Autodesk Fusion 360 part; units mm, degrees
sketch "Sketch1" plane through (0, 0, 0) normal (0, 1, 0) x (1, 0, 0)
  circle A0 centre (0, 0) radius 20
  circle A1 centre (0, 0) radius 17
  dimension "d1" = 40
  dimension "d7" = 3
extrude "Extrude1" add sketch "Sketch1" along normal blind 70 makes body 1
extrude "Extrude2" add sketch "Sketch1" along normal blind 4 contours A1 bodies 1
copy_body "Body->Comp1" bodies 1 removing the originals makes body 2 in component "tubeToolHolder02"
component "tubeToolHolder02" placed x (1, 0, 0) y (0, 1, 0) z (0, 0, 1) at (0, 0, 0)
Read the model definition and answer for the solid it produces. Units are mm, in the model's axes. A direction names the side the tool comes from. Round coordinates to 2 decimals unless told otherwise and drop trailing zeros. Write each loop counter-clockwise with the first axis right and the second up, starting at its lowest first coordinate (ties: lowest second). Pieces come first, ordered by that corner, then holes. Notation, with made-up numbers: (87, 46) -> (139, 46) arc R18 cw to (139, 59) -> close; hole circle Ø2 at (13, 85.25). An arc over 180 degrees is marked (long way). Answer in a Markdown table with one row per item. Add a question column.
1) Find section A-A, the plane z = 0. Determine the outline of the cut face in (x, y), and give its area (3 significant figures).
2) Which of the six approach directions +Z, -Z, +X, -X, +Y, -Y give full straight-line access (tool end or side, diameter ignored) to faces 4 (the face through (-9, 70, 15)), 5 (the face through (0, 4, 0))?
3) Given P1, Ø1, axis at x = -6, y = 9, coming from the -Z side; P2, Ø4, axis at y = 29, z = -10, coming from the -X side; P3, Ø17, axis at x = -4, z = 0.5, coming from the +Y side, each flat-ended and moving along its own axis, determine where each tip first touches the part or whether it passes through.
4) Find section B-B, the plane x = 0. Determine the outline of the cut face in (y, z), and give its area (3 significant figures).
5) Find section C-C, the plane y = 40. Determine the outline of the cut face in (x, z), and give its area (3 significant figures).
6) Consider line 1 (X direction, y = 56, z = 0); line 2 (Y direction, x = 14, z = -4). Determine where each line is inside the solid, lowest interval first.
7) Determine the mould class of faces 1 (the face through (9.139, 36.538, 14.334)), 2 (the face through (0, 0, 0)), 3 (the face through (-4.336, 34.51, -19.524)) for opening direction Z: pulls with the +Z half, pulls with the -Z half, needs draft (parallel to the pull), parting line crosses it, or undercut.
Findings below:
| question | item | result |
|---|---|---|
| 1 | outline | (-20, 0) -> (20, 0) -> (20, 70) -> (17, 70) -> (17, 4) -> (-17, 4) -> (-17, 70) -> (-20, 70) -> close |
| 1 | area | 556 mm² |
| 2 | face 4 | +Z, -Z, +X, -X, +Y |
| 2 | face 5 | +Y |
| 3 | P1 | z = -19.23 |
| 3 | P2 | x = -18.33 |
| 3 | P3 | y = 4 |
| 4 | outline | (0, -20) -> (70, -20) -> (70, -17) -> (4, -17) -> (4, 17) -> (70, 17) -> (70, 20) -> (0, 20) -> close |
| 4 | area | 556 mm² |
| 5 | outline | circle Ø40 at (0, 0); hole circle Ø34 at (0, 0) |
| 5 | area | 349 mm² |
| 6 | line 1 | -20 to -17, 17 to 20 |
| 6 | line 2 | 0 to 4 |
| 7 | face 1 | undercut |
| 7 | face 2 | needs draft |
| 7 | face 3 | parting line crosses it |
